from build123d import *

# Parameters (mm, degrees)
SKETCH1_R               = 30
SKETCH1_R_2             = 19
BOSS_EXTRUDE1_DEPTH     = 6
SKETCH1_R_3             = 4.8
BOSS_EXTRUDE1_2_DEPTH   = 6
EXTRUDE_THIN1_DEPTH     = 6
CIRPATTERN1_COUNT       = 2
SKETCH9_R               = 4.086461839
BOSS_EXTRUDE3_DEPTH     = 2.5
CUT_EXTRUDE2_REACH      = 44.849
SKETCH4_R               = 1.6125
CIRPATTERN2_COUNT       = 6
CUT_EXTRUDE3_DEPTH      = 43.848570725
CUT_EXTRUDE3_DEPTH_BACK = 43.848570725
CUT_EXTRUDE4_REACH      = 44.849
FILLET3_R               = 0.5


# Read off the part's stored shape, not the designer's step: Extrude-Thin1
with BuildPart() as part:
    # Sketch1 → Boss-Extrude1 (new body)
    with BuildSketch(Plane.XY):
        Circle(SKETCH1_R)
        Circle(SKETCH1_R_2, mode=Mode.SUBTRACT)
    extrude(amount=BOSS_EXTRUDE1_DEPTH)



with BuildPart() as body_2:
    # Sketch1 → Boss-Extrude1 2 (new body)
    with BuildSketch(Plane.XY):
        Circle(SKETCH1_R_3)
    extrude(amount=BOSS_EXTRUDE1_2_DEPTH)


with BuildPart() as part_1:
    add(part.part)

    add(body_2.part)  # Extrude-Thin1 merges body 2
    # Extrude-Thin1 outline → Extrude-Thin1 (add)
    with BuildSketch(Plane.XY):
        with BuildLine():
            ThreePointArc((-2.982283939, -3.76111453), (-4.633404211, -1.253620924), (-4.471841365, 1.744314996))
            add(Edge.make_bspline(
                [(-4.471841365, 1.744314996), (-4.656280132, 1.578520884), (-4.829643815, 1.39644694), (-5.268134024, 0.859774522), (-5.508550979, 0.475921884), (-6.089314004, -0.796416981), (-6.277652461, -1.775043044), (-6.156958422, -3.849228134), (-5.848111539, -4.916888286), (-4.701074788, -6.924579158), (-3.874352285, -7.841881846), (-1.772209934, -9.303379732), (-0.515534208, -9.833026737), (2.2585228, -10.322842004), (3.754003283, -10.277922339), (6.737860458, -9.516399172), (8.205073527, -8.803982666), (10.830706996, -6.729759977), (11.973176133, -5.377828677), (13.242651036, -2.985752228), (13.590862634, -2.130587863), (14.11230257, -0.33141552), (14.284853693, 0.610384541), (14.434244224, 2.54590596), (14.410872075, 3.537351035), (14.155614086, 5.530618766), (13.92398055, 6.530190205), (13.24831887, 8.495265), (12.804987465, 9.458632364), (11.711589511, 11.305878718), (11.062628134, 12.187820678), (9.57337189, 13.827874293), (8.734539676, 14.584322286), (6.890445718, 15.932212548), (5.886940321, 16.522327046), (3.747220053, 17.501569877), (2.612981166, 17.889754848), (0.253213214, 18.436226952), (-0.970201662, 18.593988054), (-2.775234189, 18.641394623), (-3.338985958, 18.630807023), (-3.904551177, 18.594474451)],
                knots=[0.013114223, 0.013114223, 0.013114223, 0.013114223, 0.03125, 0.03125, 0.0625, 0.0625, 0.125, 0.125, 0.1875, 0.1875, 0.25, 0.25, 0.3125, 0.3125, 0.375, 0.375, 0.4375, 0.4375, 0.5, 0.5, 0.53125, 0.53125, 0.5625, 0.5625, 0.59375, 0.59375, 0.625, 0.625, 0.65625, 0.65625, 0.6875, 0.6875, 0.71875, 0.71875, 0.75, 0.75, 0.78125, 0.78125, 0.8125, 0.8125, 0.826547707, 0.826547707, 0.826547707, 0.826547707], degree=3))
            ThreePointArc((-3.904551177, 18.594474451), (-13.097935775, 13.763868585), (-18.378155197, 4.821142141))
            add(Edge.make_bspline(
                [(-2.982283939, -3.76111453), (-2.900117375, -3.985308214), (-2.796401924, -4.21083352), (-2.324302177, -5.037163062), (-1.796089022, -5.632977998), (-0.42544773, -6.585905543), (0.434939841, -6.954445423), (2.351330437, -7.292822525), (3.427095408, -7.265193511), (5.581040851, -6.715475726), (6.677239672, -6.187769457), (8.63917944, -4.637857777), (9.517283547, -3.605835215), (10.495671123, -1.762255736), (10.766831426, -1.097457986), (11.173484801, 0.30565569), (11.309561474, 1.046104982), (11.427328915, 2.571913894), (11.409154422, 3.359454964), (11.205932916, 4.946378335), (11.020577877, 5.747900562), (10.477750396, 7.326644233), (10.119550016, 8.105878633), (9.233725774, 9.602438596), (8.704992436, 10.321571812), (7.489073995, 11.660610304), (6.800450018, 12.282049392), (5.283951031, 13.39049303), (4.454371448, 13.878701098), (2.6829423, 14.689395523), (1.739195133, 15.012712578), (-0.226650012, 15.467960532), (-1.25075985, 15.600322026), (-3.337683593, 15.655132061), (-4.402541801, 15.577599807), (-6.527123675, 15.202481181), (-7.588842349, 14.904507495), (-9.660915862, 14.087662981), (-10.673137841, 13.568018908), (-12.599590732, 12.316810654), (-13.515488441, 11.58412259), (-15.204366904, 9.925715954), (-15.9787504, 8.998571318), (-17.325389887, 7.006470862), (-17.903482072, 5.944264002), (-18.378155197, 4.821142141)],
                knots=[0.164583944, 0.164583944, 0.164583944, 0.164583944, 0.1875, 0.1875, 0.25, 0.25, 0.3125, 0.3125, 0.375, 0.375, 0.4375, 0.4375, 0.5, 0.5, 0.53125, 0.53125, 0.5625, 0.5625, 0.59375, 0.59375, 0.625, 0.625, 0.65625, 0.65625, 0.6875, 0.6875, 0.71875, 0.71875, 0.75, 0.75, 0.78125, 0.78125, 0.8125, 0.8125, 0.84375, 0.84375, 0.875, 0.875, 0.90625, 0.90625, 0.9375, 0.9375, 0.96875, 0.96875, 0.999171124, 0.999171124, 0.999171124, 0.999171124], degree=3))
        make_face()
    extrude_thin1 = extrude(amount=EXTRUDE_THIN1_DEPTH)

    # CirPattern1: Extrude-Thin1 ×2 about axis
    cirpattern1_axis = Axis((0, 0, 6), (0, 0, -1))
    for i in range(1, CIRPATTERN1_COUNT):
        add(extrude_thin1.rotate(cirpattern1_axis, i * 360 / CIRPATTERN1_COUNT))

    # Sketch9 → Boss-Extrude3 (add)
    with BuildSketch(Plane(origin=(0, 0, 0), x_dir=(-1, 0, 0), z_dir=(0, 0, -1))):
        with Locations(Location((0, 0, 0), (0, 0, 180))):
            Circle(SKETCH9_R)
    extrude(amount=BOSS_EXTRUDE3_DEPTH)

    # Sketch4 → Cut-Extrude2 (cut, up to next)
    with BuildSketch(Plane.XY, mode=Mode.PRIVATE) as cut_extrude2_sk1:
        with Locations(Location((-25, 0, 0), (0, 0, 180))):
            Circle(SKETCH4_R)
    cut_extrude2_tool1 = extrude(cut_extrude2_sk1.sketch, amount=CUT_EXTRUDE2_REACH, mode=Mode.PRIVATE) & part_1.part
    cut_extrude2 = cut_extrude2_tool1.solids().sort_by_distance((-25, 0, 0))[0]
    add(cut_extrude2, mode=Mode.SUBTRACT)

    # CirPattern2: Cut-Extrude2 ×6 about axis
    cirpattern2_axis = Axis((0, 0, 0), (0, 0, 1))
    for i in range(1, CIRPATTERN2_COUNT):
        add(cut_extrude2.rotate(cirpattern2_axis, i * 360 / CIRPATTERN2_COUNT), mode=Mode.SUBTRACT)

    # Sketch6 → Cut-Extrude3 (cut, two sides: drawn at the far end of the back side and taken through both)
    with BuildSketch(Plane.XY.offset(-CUT_EXTRUDE3_DEPTH_BACK)):
        with BuildLine():
            Line((-2.397915762, 2.375), (2.397915762, 2.375))
            ThreePointArc((2.397915762, 2.375), (0, -3.375), (-2.397915762, 2.375))
        make_face()
    extrude(amount=CUT_EXTRUDE3_DEPTH + CUT_EXTRUDE3_DEPTH_BACK, mode=Mode.SUBTRACT)

    # Sketch7 → Cut-Extrude4 (cut, up to next)
    with BuildSketch(Plane.XY, mode=Mode.PRIVATE) as cut_extrude4_sk1:
        with BuildLine():
            ThreePointArc((-4.471841365, 1.744314996), (-2.708070163, 3.963124524), (0, 4.8))
            ThreePointArc((0, 4.8), (-2.503483375, 3.663722045), (-4.471841365, 1.744314996))
        make_face()
    cut_extrude4_tool1 = extrude(cut_extrude4_sk1.sketch, amount=CUT_EXTRUDE4_REACH, mode=Mode.PRIVATE) & part_1.part
    # Sketch7 → Cut-Extrude4 (cut, up to next)
    with BuildSketch(Plane.XY, mode=Mode.PRIVATE) as cut_extrude4_sk2:
        with BuildLine():
            ThreePointArc((4.471841365, -1.744314996), (2.708070163, -3.963124524), (0, -4.8))
            ThreePointArc((0, -4.8), (2.503483375, -3.663722045), (4.471841365, -1.744314996))
        make_face()
    cut_extrude4_tool2 = extrude(cut_extrude4_sk2.sketch, amount=CUT_EXTRUDE4_REACH, mode=Mode.PRIVATE) & part_1.part
    add(cut_extrude4_tool1.solids().sort_by_distance((-2.531789, 3.705146, 0))[0], mode=Mode.SUBTRACT)
    add(cut_extrude4_tool2.solids().sort_by_distance((2.531789, -3.705146, 0))[0], mode=Mode.SUBTRACT)

    # Fillet3
    fillet3_edges = [part_1.edges().sort_by_distance(p)[0] for p in [
        (-3.904551177, 18.594474451, 3),
        (-2.982283939, -3.76111453, 3),
        (2.982283939, 3.76111453, 3),
        (3.904551177, -18.594474451, 3),
    ]]
    fillet(fillet3_edges, radius=FILLET3_R)


solid = part_1.part
The listing builds one solid part. Answer for the finished solid, in the listing's coordinates (mm). A direction names the side the tool comes from. Give positions to 0.01 mm unless a question says otherwise; leave off trailing zeros. Loops run counter-clockwise (first coordinate to the right, second up) from the corner with the lowest first, then second, coordinate; pieces in that order, holes last.
Item 1: Find the intervals of material crossed by line 1 along X through (y, z) = (8, 1.75); line 2 along Y through (x, z) = (12.5, 1.7); line 3 along Y through (x, z) = (-12.5, 2.8), in increasing order.
Derived:
line 1: x = -28.91 to -16.65, -9.21 to 3.56, 10.14 to 13.41, 17.23 to 28.91
line 2: y = -27.27 to -23.26, -20.04 to -12.34, -4.35 to 9.96, 14.31 to 20.04, 23.26 to 27.27
line 3: y = -27.27 to -23.26, -20.04 to -14.31, -9.96 to 4.35, 12.34 to 20.04, 23.26 to 27.27
Item 2: A cutting plane is placed at D-D (y = 0). Give the number of separate pieces and of enclosed holes in the cut face, then the cut area to 3 significant figures.
Derived:
separate pieces: 8
enclosed holes: 0
area: 162 mm2
Item 3: Each of these flat-tipped pins is pushed along its axis until it touches: pin 1 Ø5 at (x, z) = (-16, -1.5) entering from +Y; pin 2 Ø4 at (y, z) = (-11.5, 3.5) entering from +X; pin 3 Ø10 at (x, y) = (-9, -4) entering from +Z; pin 4 Ø4 at (x, z) = (-0.5, 1.5) entering from -Y. Where does it stop, or does it pass through?
Derived:
pin 1: stops at y = 26.53
pin 2: stops at x = 28.46
pin 3: stops at z = 6
pin 4: stops at y = -30
Item 4: A cutting plane is placed at B-B (z = -1.75). Give the vertices of the cut face in (x, y) (3 decimals).
Derived:
outline: circle Ø8.173 at (0, 0); hole (-2.398, 2.375) arc R3.375 ccw (long way) to (2.398, 2.375) - close
Item 5: A cutting plane is placed at A-A (y = 22). Give the vertices of the cut face in (x, z), then the cut area to 3 significant figures.
Derived:
outline: (-20.4, 0) - (-14.07, 0) - (-14.07, 6) - (-20.4, 6) - close; (-10.93, 0) - (10.93, 0) - (10.93, 6) - (-10.93, 6) - close; (14.07, 0) - (20.4, 0) - (20.4, 6) - (14.07, 6) - close
area: 207 mm2
Item 6: Determine the mould class of faces 4 (the cylindrical face through (-29.97, 1.32, 2.96)), 5 (the cylindrical face through (16.05, 10.17, 2.96)), 6 (the flat face through (0, 7, 0)) for opening direction Y: +Y half, -Y half, draft (parallel to the pull), parting line (faces both ways), or undercut.
Derived:
face 4: parting line
face 5: undercut
face 6: draft
Item 7: A cutting plane is placed at C-C (x = 25). Give the vertices of the cut face in (y, z).
Derived:
outline: (-16.58, 0) - (-1.61, 0) - (-1.61, 6) - (-16.58, 6) - close; (1.61, 0) - (16.58, 0) - (16.58, 6) - (1.61, 6) - close
Item 8: A tool of negligible diameter and unlimited length cuts with its end or side. For faces 1 (the flat face through (0, 2.375, 2)), 2 (the cylindrical face through (-3.012, -2.762, -1.232)), 3 (the flat face through (0, 3, -2.5)), from which of +Z, -Z, +X, -X, +Y, -Y can it reach the whole face along a straight path? Write none if from no direction.
Derived:
face 1: +Z, -Z
face 2: -Z
face 3: -Z, +X, -X, +Y, -Y
